Read the model definition and answer for the solid it produces. Units are mm, in the model's axes. A direction names the side the tool comes from. Coordinates: 2 decimals unless noted, no trailing zeros. Loops run counter-clockwise (first coordinate to the right, second up) from the corner with the lowest first, then second, coordinate; pieces in that order, holes last.
Q1. Flat-ended cylindrical pins translate along their axes: P1, Ø11, axis at x = -0.5, y = -29.5, coming from the +Z side; P2, Ø6, axis at x = -11.5, z = -24.5, coming from the +Y side; P3, Ø23, axis at y = -21, z = -80, coming from the -X side. Find the tip coordinate at first contact, or state that the pin passes through.
Q2. Section A-A (y = -32.5) is taken. Give the vertices of the cut face in (x, z).
Q3. Which of the six approach directions +Z, -Z, +X, -X, +Y, -Y give full straight-line access (tool end or side, diameter ignored) to faces 1 (the face through (7, -21, -85)), 2 (the face through (-7, -21, -85)), 3 (the face through (25, 0, 30)), 4 (the face through (-15, 0, 39))?
Q4. Section B-B (z = -85) is taken. Give the vertices of the cut face in (x, y), then the cut area to 3 significant figures.
Q5. Straight lines are drawn through the part: line 1 (X direction, y = 17, z = 24); line 2 (Z direction, x = -4, y = -32.5); line 3 (X direction, y = -2, z = 32.5). For each, find the intervals that lie inside material, in ascending order.
Q6. The mould has two halves that part along Z. Classify faces 5 (the face through (0, -42.5, -85)), 6 (the face through (0, 0, 10)), 7 (the face through (30, 0, 50)), 8 (the face through (-0.098, -31.393, -76.572)): pulls with the +Z half, pulls with the -Z half, needs draft (parallel to the pull), parting line crosses it, or undercut.
Q7. Section D-D (z = -58) is taken. Give the vertices of the cut face in (x, y).
Q8. Section C-C (x = 32) is taken. Give the vertices of the cut face in (y, z).
from build123d import *

# Parameters (mm, degrees)
F0_W      = 90
F0_H      = 60
F1_DEPTH  = 10
F2_W      = 10
F2_H      = 60
F3_DEPTH  = 20
F5_W      = 30
F5_H      = 60
F6_DEPTH  = 20
F4_W      = 30
F4_H      = 60
F7_DEPTH  = 20
F8_W      = 40
F8_H      = 15
F9_DEPTH  = 100
F10_W     = 14
F10_H     = 25
F11_DEPTH = 50
F12_R     = 8.5
F13_DEPTH = 52.001
F14_R     = 2


with BuildPart() as f1:
    # F0 (on Top) → F1 (new body)
    with BuildSketch(Plane.XY):
        Rectangle(F0_W, F0_H)
    extrude(amount=F1_DEPTH)

    # F2 (on face) → F3 (join)
    with BuildSketch(Plane.XY.offset(10)):
        with Locations((-40, 0)):
            Rectangle(F2_W, F2_H)
        with Locations((40, 0)):
            Rectangle(F2_W, F2_H)
    extrude(amount=F3_DEPTH)

    # F5 (on face) → F6 (join)
    with BuildSketch(Plane.XY.offset(30)):
        with Locations((30, 0)):
            Rectangle(F5_W, F5_H)
    extrude(amount=F6_DEPTH)

    # F4 (on face) → F7 (join)
    with BuildSketch(Plane.XY.offset(30)):
        with Locations((-30, 0)):
            Rectangle(F4_W, F4_H)
    extrude(amount=F7_DEPTH)

    # F8 (on face) → F9 (join)
    with BuildSketch(Plane(origin=(0, 0, 0), x_dir=(1, 0, 0), z_dir=(0, 0, -1))):
        Rectangle(F8_W, F8_H)
    extrude(amount=F9_DEPTH)

    # F10 (on face) → F11 (join)
    with BuildSketch(Plane(origin=(0, 7.5, 0), x_dir=(-1, 0, 0), z_dir=(0, 1, 0))):
        with Locations((0, -85)):
            Rectangle(F10_W, F10_H)
    extrude(amount=-F11_DEPTH)

    # F12 (on face) → F13 (cut, through all)
    with BuildSketch(Plane(origin=(-7, 0, 0), x_dir=(0, -1, 0), z_dir=(-1, 0, 0))):
        with Locations((32.5, -85)):
            Circle(F12_R)
    extrude(amount=-F13_DEPTH, mode=Mode.SUBTRACT)

    # F14
    f14_edges = [f1.edges().sort_by_distance(p)[0] for p in [
        (-20, 7.5, -50),
        (0, 7.5, -100),
        (20, 7.5, -50),
        (20, 0, -100),
        (-20, 0, -100),
        (-20, -7.5, -50),
        (20, -7.5, -50),
        (20, 0, 0),
        (0, -7.5, -100),
        (0, 30, 0),
        (45, 30, 25),
        (30, 30, 50),
        (-15, 30, 40),
        (-30, 30, 50),
        (-45, 30, 25),
        (-45, 0, 0),
        (-45, 0, 50),
        (-45, -30, 25),
        (0, -30, 0),
        (45, 0, 0),
        (45, -30, 25),
        (45, 0, 50),
        (30, -30, 50),
        (-15, -30, 40),
        (-30, -30, 50),
        (-15, 0, 50),
        (15, 0, 50),
        (-7, -25, -97.5),
        (-7, -25, -72.5),
        (7, -25, -97.5),
        (7, -25, -72.5),
        (0, 7.5, 0),
        (-20, 0, 0),
        (0, -7.5, 0),
    ]]
    fillet(f14_edges, radius=F14_R)


solid = f1.part
Numbers:
1. P1: stops at z = 10
1. P2: stops at y = 7.5
1. P3: stops at x = -7
2. outline: (-7, -95.5) arc R2 ccw to (-5, -97.5) - (5, -97.5) arc R2 ccw to (7, -95.5) - (7, -93.5) - (-7, -93.5) - close; (-7, -76.5) - (7, -76.5) - (7, -74.5) arc R2 ccw to (5, -72.5) - (-5, -72.5) arc R2 ccw to (-7, -74.5) - close
3. face 1: -Z, +X, -Y
3. face 2: -Z, -X, -Y
3. face 3: +Y, -Y
3. face 4: +Z, +Y, -Y
4. outline: (-20, -5.5) arc R2 ccw to (-18, -7.5) - (-7, -7.5) - (-7, -24) - (7, -24) - (7, -7.5) - (18, -7.5) arc R2 ccw to (20, -5.5) - (20, 5.5) arc R2 ccw to (18, 7.5) - (-18, 7.5) arc R2 ccw to (-20, 5.5) - close; (-7, -42.5) - (7, -42.5) - (7, -41) - (-7, -41) - close
4. area: 849 mm2
5. line 1: x = -45 to -35, 35 to 45
5. line 2: z = -97.5 to -93.5, -76.5 to -72.5
5. line 3: x = -45 to -15, 15 to 45
6. face 5: needs draft
6. face 6: undercut
6. face 7: pulls with the +Z half
6. face 8: undercut
7. outline: (-20, -5.5) arc R2 ccw to (-18, -7.5) - (18, -7.5) arc R2 ccw to (20, -5.5) - (20, 5.5) arc R2 ccw to (18, 7.5) - (-18, 7.5) arc R2 ccw to (-20, 5.5) - close
8. outline: (-30, 2) arc R2 ccw to (-28, 0) - (28, 0) arc R2 ccw to (30, 2) - (30, 10) - (-30, 10) - close; (-30, 30) - (30, 30) - (30, 48) arc R2 ccw to (28, 50) - (-28, 50) arc R2 ccw to (-30, 48) - close
